Geometry: final body of the model. Coordinates: model frame, mm. A direction names the side the tool comes from. Round coordinates to 2 decimals unless told otherwise and drop trailing zeros. Write each loop counter-clockwise with the first axis right and the second up, starting at its lowest first coordinate (ties: lowest second). Pieces come first, ordered by that corner, then holes. Notation, with made-up numbers: M 73.25,88 L 129.25,88 A13 ccw 129.25,110 Z; hole C 78,33.25 d2. An arc over 180 degrees is marked long. Answer as CSV lines item,"result". Start each with the question number.
Q1. Ray query, probe 1 along Z at (x, y) = (-15, 6); probe 2 along X at (y, z) = (-5, 46.5); probe 3 along Y at (x, z) = (-11, 15.5). Return the intervals inside material, ascending.
Q2. Section query A-A on z = 24. Output: boundary loops of the cut face in (x, y), and give its area (3 significant figures).
Q3. Reachability of faces 1 (the cylindrical face through (2.17, 9.76, -12.32)), 2 (the flat face through (2.13, 3.77, 95.93)), 3 (the flat face through (-2.2, 3.73, 95.93)), 4 (the flat face through (-4.33, 0, 96)) from +Z, -Z, +X, -X, +Y, -Y: full face, straight path, thin tool, end or side. Return the list, or none.
Q4. Section query C-C on x = -17.5. Output: boundary loops of the cut face in (y, z), and give its area (3 significant figures).
Q5. Section query B-B on x = 19. Output: boundary loops of the cut face in (y, z).
Q6. First-contact query: pin 1 (5 mm diameter, centred on x = -13.5, y = -1.5, fed in from -Z); pin 2 (2.5 mm diameter, centred on y = -0.5, z = 95.5, fed in from -X); pin 3 (3 mm diameter, centred on y = 16.5, z = 41.5, fed in from +X). Flat tips, straight axial feed; report the tip coordinate or a pass-through.
Autodesk Inventor part; units mm, degrees
ref_plane "YZ Plane" through (0, 0, 0) normal (1, 0, 0) x (0, 1, 0)
ref_plane "XZ Plane" through (0, 0, 0) normal (0, 1, 0) x (-1, 0, 0)
ref_plane "XY Plane" through (0, 0, 0) normal (0, 0, 1) x (1, 0, 0)
sketch "Boceto1" plane through (0, 0, 0) normal (0, 0, 1) x (1, 0, 0)
  circle A0 centre (0, 0) radius 21.75
  arc A1 (1.304413, 21.71085) -> (0, 23.055) centre (0, 21.75) ccw
  arc A2 (0, 23.055) -> (-1.304413, 21.71085) centre (0, 21.75) ccw
  line L0 (0, -21.75) -> (0, -23.25)
  arc A3 (0, -23.25) -> (1.499108, -21.698276) centre (0, -21.75) ccw
  arc A4 (-1.499108, -21.698276) -> (0, -23.25) centre (0, -21.75) ccw
  line L1 (21.75, 0) -> (23.055, 0)
  line L2 (-21.75, 0) -> (-23.25, 0)
  arc A5 (-21.698276, 1.499108) -> (-21.698276, -1.499108) centre (-21.75, 0) ccw
  arc A6 (21.71085, -1.304413) -> (21.71085, 1.304413) centre (21.75, 0) ccw
  dimension "d0" = 43.5
  dimension "d2" = 1.5
  dimension "d4" = 1.5
extrude "Extrusión1" add sketch "Boceto1" along normal blind 81
sketch "Boceto2" plane through (0, 0, 81) normal (0, 0, 1) x (1, 0, 0)
  line L0 (0, 5) -> (4.330127, 2.5)
  line L1 (4.330127, 2.5) -> (4.330127, -2.5)
  line L2 (4.330127, -2.5) -> (0, -5)
  line L3 (0, -5) -> (-4.330127, -2.5)
  line L4 (-4.330127, -2.5) -> (-4.330127, 2.5)
  line L5 (-4.330127, 2.5) -> (0, 5)
  point P0 (0, 0)
  point P1 (0, 0)
extrude "Extrusión2" add sketch "Boceto2" along normal blind 20
sketch "Boceto10" plane through (0, 0, 0) normal (0, 0, -1) x (-1, 0, 0)
  circle A0 centre (0, 0) radius 7.5
  dimension "d37" = 15
extrude "Extrusión9" add sketch "Boceto10" along normal blind 25
sketch "Boceto12" plane through (0, 0, 0) normal (0, 0, -1) x (-1, 0, 0)
  circle A0 centre (0, 0) radius 10
  dimension "d40" = 20
extrude "Extrusión10" add sketch "Boceto12" along normal blind 25
sketch "Boceto20" plane through (0, 0, 81) normal (0, 0, 1) x (1, 0, 0)
  circle A0 centre (0, 0) radius 15
  dimension "d61" = 30
ref_plane "Plano de trabajo1" through (0, 0, 91) normal (0, 0, 1) x (1, 0, 0)
sketch "Boceto21" plane through (0, 0, 91) normal (0, 0, 1) x (1, 0, 0)
  line L0 (4.330127, 2.5) -> (4.330127, -2.5)
  circle A0 centre (0, 0) radius 5
sketch "Boceto20 outline for Solevación1" plane through (0, 0, 81) normal (0, 0, 1) x (1, 0, 0)
  circle A0 centre (0, 0) radius 15
sketch "Boceto21 outline for Solevación1" plane through (0, 0, 91) normal (0, 0, 1) x (1, 0, 0)
  circle A0 centre (0, 0) radius 5
loft "Solevación1" add profiles "Boceto20 outline for Solevación1", "Boceto21 outline for Solevación1"
sketch "Boceto22" plane through (0, 0, 81) normal (0, 0, 1) x (1, 0, 0)
  arc A0 (1.304413, 21.71085) -> (-1.304413, 21.71085) centre (0, 21.75) ccw
  arc A1 (1.304413, 21.71085) -> (-1.304413, 21.71085) centre (0, 21.749554) ccw
  arc A2 (21.71085, -1.304413) -> (21.71085, 1.304413) centre (21.75, 0) ccw
  arc A3 (21.71085, -1.304413) -> (21.71085, 1.304413) centre (21.749554, 0) ccw
  arc A4 (-1.499108, -21.698276) -> (1.499108, -21.698276) centre (0, -21.75) ccw
  arc A5 (-1.499108, -21.698276) -> (1.499108, -21.698276) centre (0, -21.749411) ccw
  arc A6 (-21.698276, 1.499108) -> (-21.698276, -1.499108) centre (-21.75, 0) ccw
  arc A7 (-21.685394, 1.49099) -> (-21.698276, -1.499108) centre (-21.753079, -0.003795) ccw
  arc A8 (-21.698276, 1.499108) -> (-21.698276, -1.499108) centre (-1.222086, 0) ccw
  arc A9 (1.304413, 21.71085) -> (-1.304413, 21.71085) centre (0, -0.250446) ccw
  arc A10 (21.71085, -1.304413) -> (21.71085, 1.304413) centre (-0.250446, 0) ccw
  arc A11 (-1.499108, -21.698276) -> (1.499108, -21.698276) centre (0, 0.250589) ccw
  point P0 (0, 0)
sketch "Boceto22 outline for Extrusión16" plane through (0, 0, 81) normal (0, 0, 1) x (1, 0, 0)
  arc A0 (-1.304413, 21.71085) -> (1.304413, 21.71085) centre (0, -0.250446) cw
  arc A1 (1.304413, 21.71085) -> (-1.304413, 21.71085) centre (0, 21.75) ccw
  arc A2 (21.71085, 1.304413) -> (21.71085, -1.304413) centre (-0.250446, 0) cw
  arc A3 (21.71085, -1.304413) -> (21.71085, 1.304413) centre (21.75, 0) ccw
  arc A4 (-21.698276, -1.499108) -> (-21.698276, 1.499108) centre (-1.222086, 0) cw
  arc A5 (-21.698276, 1.499108) -> (-21.698276, -1.499108) centre (-21.75, 0) ccw
  arc A6 (1.499108, -21.698276) -> (-1.499108, -21.698276) centre (0, 0.250589) cw
  arc A7 (-1.499108, -21.698276) -> (1.499108, -21.698276) centre (0, -21.75) ccw
extrude "Extrusión16" cut sketch "Boceto22 outline for Extrusión16" against normal blind 211
properties part number "eix bobina"
Entries:
1,probe 1,"z = 0 to 81"
1,probe 2,"x = -21.17 to 21.17"
1,probe 3,"y = -18.76 to 18.76"
2,outline,"M -21.7,-1.5 A21.75 ccw -1.5,-21.7 A22 ccw 1.5,-21.7 A21.75 ccw 21.71,-1.3 A22 ccw 21.71,1.3 A21.75 ccw 1.3,21.71 A22 ccw -1.3,21.71 A21.75 ccw -21.7,1.5 A20.53 ccw Z"
2,area,"1,490 mm^2"
3,face 1,"-Z"
3,face 2,"+Z, +X, +Y"
3,face 3,"+Z, -X, +Y"
3,face 4,"+Z, -X, +Y, -Y"
4,outline,"M -12.92,0 L 12.92,0 L 12.92,81 L -12.92,81 Z"
4,area,"2,090 mm^2"
5,outline,"M -10.59,0 L 10.59,0 L 10.59,81 L -10.59,81 Z"
6,pin 1,"stops at z = 0"
6,pin 2,"stops at x = -4.33"
6,pin 3,"stops at x = 15.75"
